```python
from build123d import *

# Parameters (mm, degrees)
SKETCH1_R  = 3.8
BASE_DEPTH = 2.54


with BuildPart() as part:
    # Sketch1 → Base (new body)
    with BuildSketch(Plane.XY):
        with BuildLine():
            Line((-18, -6.258565559), (-18, 5.741434441))
            Line((-18, 5.741434441), (-6.7, 5.741434441))
            ThreePointArc((-6.7, 5.741434441), (0, 8.823495307), (6.7, 5.741434441))
            Line((6.7, 5.741434441), (18, 5.741434441))
            Line((18, 5.741434441), (18, -6.258565559))
            Line((18, -6.258565559), (6.7, -6.258565559))
            Line((6.7, -6.258565559), (6.7, -8.798565559))
            Line((6.7, -8.798565559), (-6.7, -8.798565559))
            Line((-6.7, -8.798565559), (-6.7, -6.258565559))
            Line((-6.7, -6.258565559), (-18, -6.258565559))
        make_face()
        with Locations((-10.5, -0.258565559)):
            Circle(SKETCH1_R, mode=Mode.SUBTRACT)
        with Locations(Location((10.5, -0.258565559, 0), (0, 0, 180))):
            Circle(SKETCH1_R, mode=Mode.SUBTRACT)
        with BuildLine():
            ThreePointArc((0.997445717, 6.178571429), (0, -6.258565559), (-0.997445717, 6.178571429))
            ThreePointArc((-0.997445717, 6.178571429), (0, 7.25), (0.997445717, 6.178571429))
        make_face(mode=Mode.SUBTRACT)
    extrude(amount=BASE_DEPTH)


solid = part.part
```
Design review of the part built by this model. Coordinates are the model's own, in mm. A direction names the side the tool comes from. Coordinates: 2 decimals unless noted, no trailing zeros. Order: outer loops, then holes, each group sorted by start corner. A loop starts at its lowest first (then second) coordinate and runs counter-clockwise, first axis right, second up. Notation, with made-up numbers: (30.25, -3) -> (71.25, -3) arc R14 cw to (71.25, 18) -> close; hole circle Ø10 at (32.25, 83.5). An arc over 180 degrees is marked (long way). One line per item, written item: value. Start each with the question number.
Q1. For probe 1 along Y at (x, z) = (-10.5, 0.55); probe 2 along X at (y, z) = (0, 1.4); probe 3 along X at (y, z) = (-2, 1.8), list the stretches that pass through material, from the lowest coordinate up.
Q2. Take a section at D-D, the plane z = 2.05. State the section outline as (x, y) points.
Q3. Tool access review of faces 1 (the flat face through (12, 5.741, 1)), 2 (the flat face through (-12, 5.741, 1)), 3 (the flat face through (6.7, -8, 1)): name each direction out of +Z, -Z, +X, -X, +Y, -Y from which nothing blocks a thin tool from reaching the whole face with its end or side.
Q4. Mouldability with a two-part tool opening along X and no side actions: class faces 4 (the cylindrical face through (-0.107, 8.823, 1.252)), 5 (the cylindrical face through (-14.296, -0.091, 1.252)), 6 (the flat face through (0, -8.799, 1)) as pulls with the +X half, pulls with the -X half, needs draft (parallel to the pull), parting line crosses it, or undercut.
Q5. Insertion check: pin 1 Ø3 at (x, y) = (-13, -7) entering from +Z; pin 2 Ø1.3 at (y, z) = (-7, 1.5) entering from -X; pin 3 Ø0.8 at (y, z) = (-7.5, 1.5) entering from +X; pin 4 Ø0.8 at (x, z) = (14, 1.5) entering from +Y. Each pin has a flat end and moves straight along its axis. Give the tip position at first contact, or say it passes through.
Q6. Take a section at B-B, the plane y = -3.5. State the section outline as (x, z) points, then the cut area to 3 significant figures.
Q7. Take a section at A-A, the plane x = 0. State the section outline as (y, z) points, then the cut area to 3 significant figures.
Q8. Take a section at C-C, the plane y = -5.75. State the section outline as (x, z) points.
Values follow:
1. probe 1: y = -6.26 to -4.06, 3.54 to 5.74
1. probe 2: x = -18 to -14.29, -6.71 to -6.26, 6.26 to 6.71, 14.29 to 18
1. probe 3: x = -18 to -13.88, -7.12 to -5.93, 5.93 to 7.12, 13.88 to 18
2. outline: (-18, -6.26) -> (-6.7, -6.26) -> (-6.7, -8.8) -> (6.7, -8.8) -> (6.7, -6.26) -> (18, -6.26) -> (18, 5.74) -> (6.7, 5.74) arc R8.82 ccw to (-6.7, 5.74) -> (-18, 5.74) -> close; hole circle Ø7.6 at (-10.5, -0.26); hole (-1, 6.18) arc R6.26 ccw (long way) to (1, 6.18) arc R1 ccw (long way) to start; hole circle Ø7.6 at (10.5, -0.26)
3. face 1: +Z, -Z, +X, +Y
3. face 2: +Z, -Z, -X, +Y
3. face 3: +Z, -Z, +X, -Y
4. face 4: parting line crosses it
4. face 5: undercut
4. face 6: needs draft
5. pin 1: stops at z = 2.54
5. pin 2: stops at x = -6.7
5. pin 3: stops at x = 6.7
5. pin 4: stops at y = 5.74
6. outline: (-18, 0) -> (-12.48, 0) -> (-12.48, 2.54) -> (-18, 2.54) -> close; (-8.52, 0) -> (-5.19, 0) -> (-5.19, 2.54) -> (-8.52, 2.54) -> close; (5.19, 0) -> (8.52, 0) -> (8.52, 2.54) -> (5.19, 2.54) -> close; (12.48, 0) -> (18, 0) -> (18, 2.54) -> (12.48, 2.54) -> close
6. area: 44.9 mm2
7. outline: (-8.8, 0) -> (-6.26, 0) -> (-6.26, 2.54) -> (-8.8, 2.54) -> close; (7.25, 0) -> (8.82, 0) -> (8.82, 2.54) -> (7.25, 2.54) -> close
7. area: 10.4 mm2
8. outline: (-18, 0) -> (-2.47, 0) -> (-2.47, 2.54) -> (-18, 2.54) -> close; (2.47, 0) -> (18, 0) -> (18, 2.54) -> (2.47, 2.54) -> close
